Verification items for the finished model (mm, model axes). Round coordinates to 2 decimals unless told otherwise and drop trailing zeros. Order: outer loops, then holes, each group sorted by start corner. A loop starts at its lowest first (then second) coordinate and runs counter-clockwise, first axis right, second up. Notation, with made-up numbers: (17, 4) -> (52, 4) arc R13 cw to (52, 23) -> close; hole circle Ø11 at (13, 24.5). An arc over 180 degrees is marked (long way). Return JSON: item names as keys, results as strings. Group by question number.
Item 1: Sectioned sample at C-C on z = 4. Give the number of separate pieces and of enclosed holes in the cut face, plus the area to 3 significant figures.
Item 2: Depth check by flat-ended pin: pin 1 Ø14.5 at (x, y) = (144.46, 754.06) entering from +Z. Enter the tip coordinate at first touch or a pass-through.
Item 3: Sectioned sample at B-B on y = 698.5. Record the cut outline in (x, z), plus the area to 3 significant figures.
Item 4: Scan lines: probe 1 along Y at (x, z) = (144, 4.4); probe 2 along Y at (x, z) = (36, 5.05); probe 3 along Y at (x, z) = (38.1, 3.25). Record each from-to range of solid material in increasing order. Write a range as from..to.
Item 5: Sectioned sample at A-A on x = 38.1. Record the cut outline in (y, z).
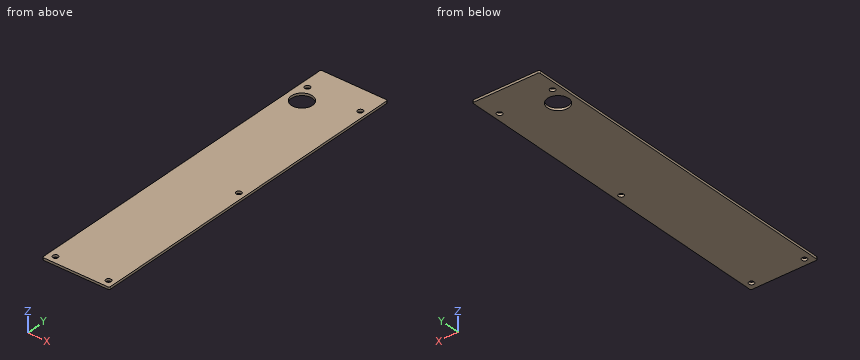
```python
from build123d import *

# Parameters (mm, degrees)
SKETCH1_W           = 160.3375
SKETCH1_H           = 814.3875
BOSS_EXTRUDE1_DEPTH = 5.588
FILLET1_R           = 3.175
SKETCH2_R           = 6.35
CUT_EXTRUDE1_DEPTH  = 6.35
SKETCH3_R           = 25.4
CUT_EXTRUDE2_DEPTH  = 831.039962777


with BuildPart() as part:
    # Sketch1 → Boss-Extrude1 (new body)
    with BuildSketch(Plane.XY):
        with Locations((80.16875, 407.19375)):
            Rectangle(SKETCH1_W, SKETCH1_H)
    extrude(amount=BOSS_EXTRUDE1_DEPTH)

    # Fillet1
    fillet1_edges = [part.edges().sort_by_distance(p)[0] for p in [
        (0, 814.3875, 2.794),
        (160.3375, 814.3875, 2.794),
        (160.3375, 0, 2.794),
        (0, 0, 2.794),
    ]]
    fillet(fillet1_edges, radius=FILLET1_R)

    # Sketch2 → Cut-Extrude1 (cut)
    with BuildSketch(Plane.XY.offset(5.588)):
        with Locations((17.4625, 754.0625)):
            Circle(SKETCH2_R)
        with Locations((144.4625, 754.0625)):
            Circle(SKETCH2_R)
        with Locations((17.4625, 17.4625)):
            Circle(SKETCH2_R)
        with Locations((144.4625, 17.4625)):
            Circle(SKETCH2_R)
        with Locations((144.4625, 398.4625)):
            Circle(SKETCH2_R)
    extrude(amount=-CUT_EXTRUDE1_DEPTH, mode=Mode.SUBTRACT)

    # Sketch3 → Cut-Extrude2 (cut, through all)
    with BuildSketch(Plane.XY.offset(5.588)):
        with Locations((38.1, 712.7875)):
            Circle(SKETCH3_R)
    extrude(amount=-CUT_EXTRUDE2_DEPTH, mode=Mode.SUBTRACT)


solid = part.part
```
Recorded:
{
 "1": {"separate pieces": "1", "enclosed holes": "6", "area": "128,000 mm²"},
 "2": {"pin 1": "z = 5.59"},
 "3": {"outline": "(0, 0) -> (17.1, 0) -> (17.1, 5.59) -> (0, 5.59) -> close; (59.1, 0) -> (160.34, 0) -> (160.34, 5.59) -> (59.1, 5.59) -> close", "area": "661 mm²"},
 "4": {"probe 1": "0..11.13, 23.8..392.13, 404.8..747.73, 760.4..814.39", "probe 2": "0..687.47, 738.1..814.39", "probe 3": "0..687.39, 738.19..814.39"},
 "5": {"outline": "(0, 0) -> (687.39, 0) -> (687.39, 5.59) -> (0, 5.59) -> close; (738.19, 0) -> (814.39, 0) -> (814.39, 5.59) -> (738.19, 5.59) -> close"}
}
